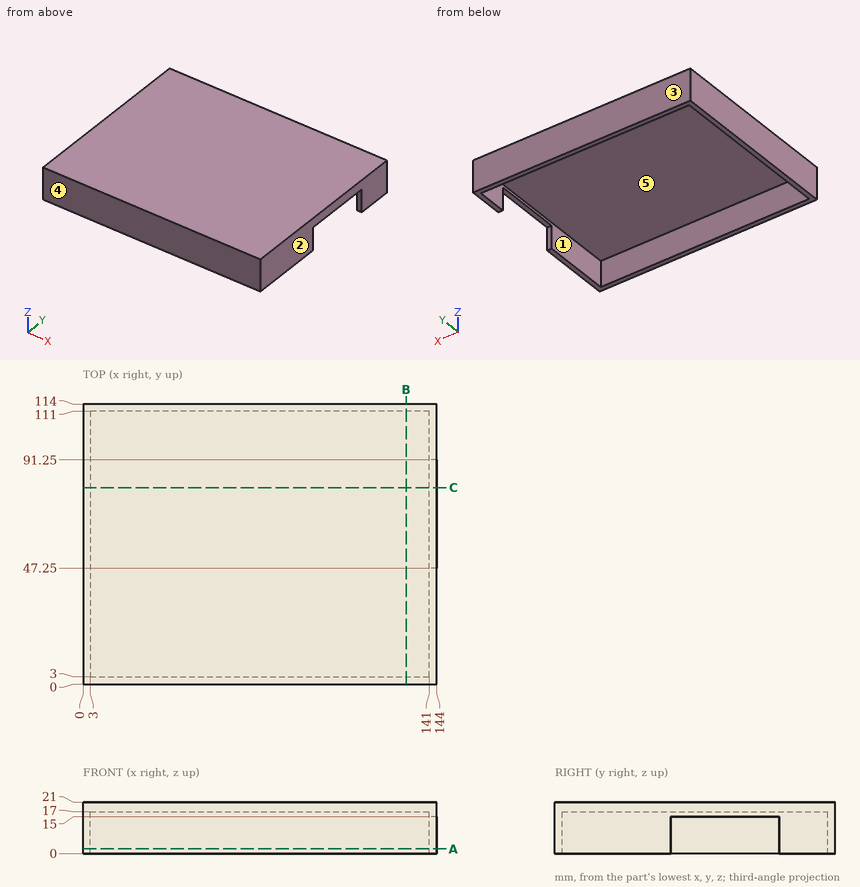
Design review of the part shown in the three views and the two pictorial views. Dimensions are in mm from the part's minimum x, y and z. A direction names the side the tool comes from. Round coordinates to 2 decimals unless told otherwise and drop trailing zeros. Loops run counter-clockwise (first coordinate to the right, second up) from the corner with the lowest first, then second, coordinate; pieces in that order, holes last. Notation, with made-up numbers: (27.25, 79) -> (52.25, 79) arc R29 cw to (52.25, 106) -> close; hole circle Ø5 at (88.25, 5). An arc over 180 degrees is marked (long way). Answer as a JSON object with one key per item and string values. Group by question number.
1) For pin 1 Ø3 at (x, y) = (47, 54.5) entering from -Z; pin 2 Ø1.5 at (x, y) = (143, 76.5) entering from -Z; pin 3 Ø1.5 at (y, z) = (84.5, 12) entering from +X, all flat-tipped, find the tip position at first contact; note any pin that passes through.
2) For line 1 (Y direction, x = 127.5, z = 9.25); line 2 (X direction, y = 42.5, z = 11); line 3 (Z direction, x = 132, y = 95), list the stretches that pass through material, from the lowest coordinate up. Write a range as [from, to].
3) We need section A-A on z = 2. Write out the cut boundary in (x, y), then the cut area to 3 significant figures.
4) We need section C-C on y = 80. Write out the cut boundary in (x, z), then the cut area to 3 significant figures.
5) For the marked faces 4 and 5, list the 3-axis set-ups (+Z, -Z, +X, -X, +Y, -Y) from which the entire face can be reached by the end or side of a thin tool; tool diameter is ignored.
6) Mouldability with a two-part tool opening along Y and no side actions: class the marked faces 1, 2 and 3 as released by +Y, released by -Y, zero draft, split by the parting line, or undercut.
7) We need section B-B on x = 131.5. Write out the cut boundary in (y, z).
Result set:
{
 "1": {"pin 1": "z = 17", "pin 2": "z = 15", "pin 3": "x = 3"},
 "2": {"line 1": "[0, 3], [111, 114]", "line 2": "[0, 3], [141, 144]", "line 3": "[17, 21]"},
 "3": {"outline": "(0, 0) -> (144, 0) -> (144, 47.25) -> (141, 47.25) -> (141, 3) -> (3, 3) -> (3, 111) -> (141, 111) -> (141, 91.25) -> (144, 91.25) -> (144, 114) -> (0, 114) -> close", "area": "1,380 mm²"},
 "4": {"outline": "(0, 0) -> (3, 0) -> (3, 17) -> (141, 17) -> (141, 15) -> (144, 15) -> (144, 21) -> (0, 21) -> close", "area": "633 mm²"},
 "5": {"face 4": "+Z, -Z, +X, -X, -Y", "face 5": "-Z"},
 "6": {"face 1": "undercut", "face 2": "zero draft", "face 3": "released by +Y"},
 "7": {"outline": "(0, 0) -> (3, 0) -> (3, 17) -> (111, 17) -> (111, 0) -> (114, 0) -> (114, 21) -> (0, 21) -> close"}
}
